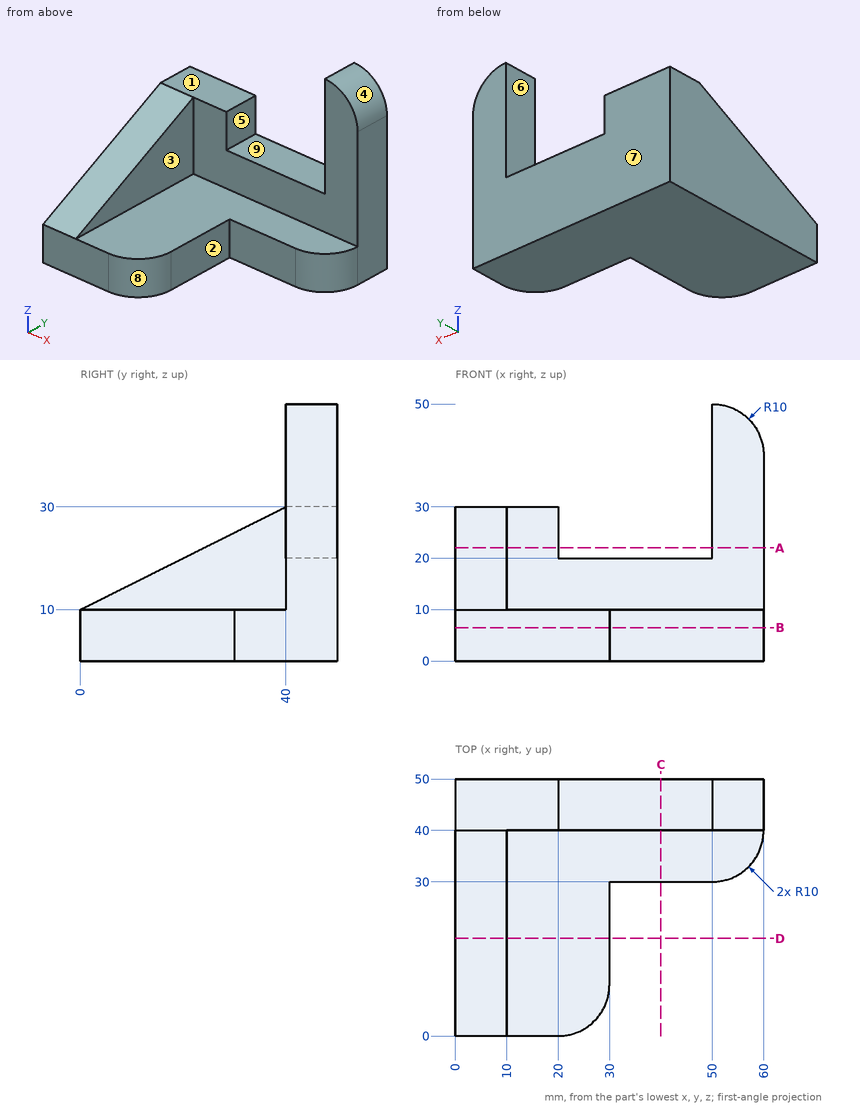
The figure shows three views and two pictorial views of one solid part (mm, origin at its lowest corner). Answer the questions. A direction names the side the tool comes from. Round coordinates to 2 decimals unless told otherwise and drop trailing zeros. Loops run counter-clockwise (first coordinate to the right, second up) from the corner with the lowest first, then second, coordinate; pieces in that order, holes last. Notation, with made-up numbers: (14, 29.25) - (18, 29.25) arc R31 cw to (18, 64.25) - close; hole circle Ø1 at (-4, 55). An arc over 180 degrees is marked (long way). Use one line per item in the form item = value. Start each with the question number.
(1) Determine the mould class of the marked faces 6, 7, 8 and 9 for opening direction X: +X half, -X half, draft (parallel to the pull), parting line (faces both ways), or undercut.
(2) Consider line 1 (X direction, y = 29.5, z = 24); line 2 (Y direction, x = 54, z = 29). Determine where each line is inside the solid, lowest interval first.
(3) Flat-ended cylindrical pins translate along their axes: P1, Ø11, axis at x = 43.5, z = 5, coming from the -Y side; P2, Ø2, axis at x = 52, y = 33, coming from the +Z side; P3, Ø3, axis at x = 9.5, y = 47.5, coming from the +Z side; P4, Ø6, axis at x = 24, z = 34, coming from the +Y side. Find the tip coordinate at first contact, or state that the pin passes through.
(4) Which of the six approach directions +Z, -Z, +X, -X, +Y, -Y give full straight-line access (tool end or side, diameter ignored) to the marked faces 1, 2, 3, 4 and 5?
(5) Find section D-D on y = 19. Determine the outline of the cut face in (x, z).
(6) Find section A-A on z = 22. Determine the outline of the cut face in (x, y).
(7) Find section B-B on z = 6.5. Determine the outline of the cut face in (x, y).
(8) Find section C-C on x = 40. Determine the outline of the cut face in (y, z).
Answer list:
q1.face_6 = undercut
q1.face_7 = draft
q1.face_8 = +X half
q1.face_9 = undercut
q2.line_1 = 0 to 10
q2.line_2 = 40 to 50
q3.P1 = 30
q3.P2 = 10
q3.P3 = 30
q3.P4 = through
q4.face_1 = +Z, -X, +Y, -Y
q4.face_2 = +Z, -Z, +X, -Y
q4.face_3 = +Z, +X, -Y
q4.face_4 = +Z, +X, +Y, -Y
q4.face_5 = +Z, +Y, -Y
q5.outline = (0, 0) - (30, 0) - (30, 10) - (10, 10) - (10, 19.5) - (0, 19.5) - close
q6.outline = (0, 24) - (10, 24) - (10, 40) - (20, 40) - (20, 50) - (0, 50) - close; (50, 40) - (60, 40) - (60, 50) - (50, 50) - close
q7.outline = (0, 0) - (20, 0) arc R10 ccw to (30, 10) - (30, 30) - (50, 30) arc R10 ccw to (60, 40) - (60, 50) - (0, 50) - close
q8.outline = (30, 0) - (50, 0) - (50, 20) - (40, 20) - (40, 10) - (30, 10) - close
